```python
from build123d import *

# Parameters (mm, degrees)
CROQUIS1_R              = 1.7272
CROQUIS1_R_2            = 2.5527
SALIENTE_EXTRUIR1_DEPTH = 0.79375


with BuildPart() as part:
    # Croquis1 → Saliente-Extruir1 (new, symmetric)
    with BuildSketch(Plane.XY):
        with BuildLine():
            ThreePointArc((-15.613365943, 2.50453349), (-16.5481, 0), (-15.613365943, -2.50453349))
            Line((-15.613365943, -2.50453349), (-9.525, -9.525))
            Line((-9.525, -9.525), (9.525, -9.525))
            Line((9.525, -9.525), (15.613365943, -2.50453349))
            ThreePointArc((15.613365943, -2.50453349), (16.5481, 0), (15.613365943, 2.50453349))
            Line((15.613365943, 2.50453349), (9.525, 9.525))
            Line((9.525, 9.525), (-9.525, 9.525))
            Line((-9.525, 9.525), (-15.613365943, 2.50453349))
        make_face()
        with Locations((-6.1976, -6.35)):
            Circle(CROQUIS1_R, mode=Mode.SUBTRACT)
        with Locations((6.5024, -6.35)):
            Circle(CROQUIS1_R, mode=Mode.SUBTRACT)
        with Locations((-12.7254, 0)):
            Circle(CROQUIS1_R_2, mode=Mode.SUBTRACT)
        with Locations((-6.1976, 6.35)):
            Circle(CROQUIS1_R, mode=Mode.SUBTRACT)
        with Locations((6.5024, 6.35)):
            Circle(CROQUIS1_R, mode=Mode.SUBTRACT)
        with Locations((12.7254, 0)):
            Circle(CROQUIS1_R_2, mode=Mode.SUBTRACT)
    extrude(amount=SALIENTE_EXTRUIR1_DEPTH, both=True)


solid = part.part
```
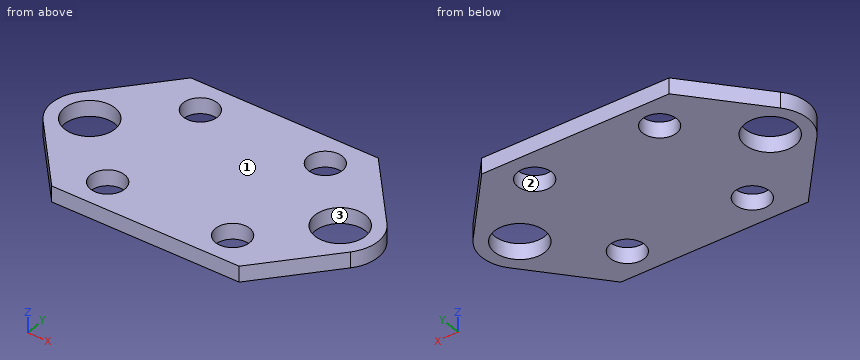
Geometry: final body of the model. Coordinates: model frame, mm. Face numbers are marked on the shaded views. Round coordinates to 2 decimals unless told otherwise and drop trailing zeros. Loops run counter-clockwise (first coordinate to the right, second up) from the corner with the lowest first, then second, coordinate; pieces in that order, holes last.
Item 1: Section C-C, the plane z = -0.05. Output: boundary loops of the cut face in (x, y) (3 decimals), plus the area to 3 significant figures.
Checked values:
outline: (-15.613, -2.505) - (-9.525, -9.525) - (9.525, -9.525) - (15.613, -2.505) arc R3.823 ccw to (15.613, 2.505) - (9.525, 9.525) - (-9.525, 9.525) - (-15.613, 2.505) arc R3.823 ccw to start; hole circle Ø5.105 at (-12.725, 0); hole circle Ø3.454 at (-6.198, -6.35); hole circle Ø3.454 at (-6.198, 6.35); hole circle Ø3.454 at (6.502, -6.35); hole circle Ø3.454 at (6.502, 6.35); hole circle Ø5.105 at (12.725, 0)
area: 437 mm2
Item 2: Section A-A, the plane x = 12. Output: boundary loops of the cut face in (y, z), plus the area to 3 significant figures.
Checked values:
outline: (-6.67, -0.79) - (-2.45, -0.79) - (-2.45, 0.79) - (-6.67, 0.79) - close; (2.45, -0.79) - (6.67, -0.79) - (6.67, 0.79) - (2.45, 0.79) - close
area: 13.4 mm2
Item 3: Contact query for a flat-ended pin moving along its axis: P1, Ø3, axis at x = 12.73, y = 0, coming from the -Z side. Output: stop coordinate, or through.
Checked values:
P1: passes through
Item 4: Section B-B, the plane y = 0. Output: boundary loops of the cut face in (x, z).
Checked values:
outline: (-16.55, -0.79) - (-15.28, -0.79) - (-15.28, 0.79) - (-16.55, 0.79) - close; (-10.17, -0.79) - (10.17, -0.79) - (10.17, 0.79) - (-10.17, 0.79) - close; (15.28, -0.79) - (16.55, -0.79) - (16.55, 0.79) - (15.28, 0.79) - close
Item 5: Section D-D, the plane x = -7.5. Output: boundary loops of the cut face in (y, z) (3 decimals), plus the area to 3 significant figures.
Checked values:
outline: (-9.525, -0.794) - (-7.484, -0.794) - (-7.484, 0.794) - (-9.525, 0.794) - close; (-5.216, -0.794) - (5.216, -0.794) - (5.216, 0.794) - (-5.216, 0.794) - close; (7.484, -0.794) - (9.525, -0.794) - (9.525, 0.794) - (7.484, 0.794) - close
area: 23.0 mm2
Item 6: Mould query, pull axis Y, two halves, no side actions, for the marked faces 1, 2 and 3. Classes: released by +Y, released by -Y, zero draft, split by the parting line, or undercut.
Checked values:
face 1: zero draft
face 2: undercut
face 3: undercut
Item 7: Line query: L1, parallel to X at y = 7, z = 0.4; L2, parallel to X at y = -1.25, z = -0.3; L3, parallel to Y at x = -7.5, z = -0.7 (3 decimals). Output: solid intervals per line, ascending.
Checked values:
L1: x = -11.71 to -7.8, -4.6 to 4.9, 8.1 to 11.71
L2: x = -16.34 to -14.95, -10.5 to 10.5, 14.95 to 16.34
L3: y = -9.525 to -7.484, -5.216 to 5.216, 7.484 to 9.525
